Solid Edge part; units mm, degrees
sketch "Sketch1" plane through (0, 0, 0) normal (0, 0, 1) x (1, 0, 0)
  line L0 (0.4577, 18.6268) -> (0.4577, 14.5625)
  line L1 (0.4577, 14.5625) -> (1.4, 14.5625)
  line L2 (1.4, 14.5625) -> (1.4, 18.192)
  arc A0 (1.4, 18.192) -> (1.603, 18.395) centre (1.603, 18.192) cw
  line L3 (1.603, 18.395) -> (6.097, 18.395)
  line L4 (6.097, 18.395) -> (6.097, 19.3373)
  line L5 (6.097, 19.3373) -> (1.1682, 19.3373)
  arc A1 (1.1682, 19.3373) -> (0.4577, 18.6268) centre (1.1682, 18.6268) ccw
revolve "RevolvedProtrusion1" add sketch "Sketch1" angle 360 about axis through (7, 0, 0) along (-1, 0, 0)
properties part number "TRAB00250"
Can you work these out from the model? Positions are in its coordinate system, mm. A direction names the side the tool comes from. Give positions to 0.01 mm unless a question says otherwise; leave off trailing zeros. Write each loop counter-clockwise with the first axis right and the second up, starting at its lowest first coordinate (ties: lowest second). Pieces come first, ordered by that corner, then holes. Notation, with made-up numbers: (54.25, -23.75) -> (103.25, -23.75) arc R23 cw to (103.25, 5.25) -> close; hole circle Ø7 at (30.25, 87.5). An arc over 180 degrees is marked (long way). Answer as a JSON object with one key per item and string values. Group by question number.
Item 1: For faces 1 (the face through (1.4, -14, -5)), 2 (the face through (6.097, 10, 16)), which set-ups out of +Z, -Z, +X, -X, +Y, -Y let a thin tool reach every point of the face, with its end or its side?
Item 2: We'd pull the mould along Y, two halves only. Please class faces 3 (the face through (3.88, 9.89, 15.51)), 4 (the face through (0.458, -11, 10)), 5 (the face through (3.598, -4.192, 18.877)): +Y half, -Y half, draft (parallel to the pull), parting line (faces both ways), or undercut.
Item 3: Suppose I cut it at C-C (x = 4.3). Please give me the cut outline in (y, z) (3 decimals).
Item 4: I'm going to push flat-ended pins straight in: P1, Ø2, axis at x = 1.5, z = 6.5, coming from the +Y side; P2, Ø22, axis at y = 0, z = 0, coming from the -X side; P3, Ø1, axis at x = 4, z = -5.5, coming from the -Y side. Where does each tip first touch, or does it pass through?
Item 5: Please list where these lines run through material, in increasing order: line 1 (Y direction, x = 1.05, z = 0); line 2 (Z direction, x = 3.95, y = 0) (3 decimals). Write a range as [from, to].
Findings:
{
 "1": {"face 1": "+X", "face 2": "+Z, -Z, +X, +Y, -Y"},
 "2": {"face 3": "undercut", "face 4": "draft", "face 5": "parting line"},
 "3": {"outline": "circle Ø38.675 at (0, 0); hole circle Ø36.79 at (0, 0)"},
 "4": {"P1": "stops at y = 18.54", "P2": "passes through", "P3": "stops at y = -18.68"},
 "5": {"line 1": "y = [-19.33, -14.56], [14.56, 19.33]", "line 2": "z = [-19.337, -18.395], [18.395, 19.337]"}
}
